```python
from build123d import *

# Parameters (mm, degrees)
SKETCH_1_R      = 3.4
SKETCH_1_W      = 10
SKETCH_1_H      = 10
EXTRUDE_1_DEPTH = 1000


with BuildPart() as part:
    # Эскиз1 → Бобышка-Вытянуть1 (new body)
    with BuildSketch(Plane.XY):
        with BuildLine():
            Line((-20, 27), (-20, 40))
            Line((-20, 40), (-7, 40))
            Line((-7, 40), (-4.1, 40))
            Line((-4.1, 40), (-4.1, 37.1))
            Line((-4.1, 37.1), (-7, 37.1))
            Line((-7, 37.1), (-7, 28.6))
            Line((-7, 28.6), (-4.582423707, 28.6))
            ThreePointArc((-4.582423707, 28.6), (-4.3976478, 28.476536686), (-4.44100235, 28.258578644))
            Line((-4.44100235, 28.258578644), (-5.571973038, 27.127607956))
            Line((-5.571973038, 27.127607956), (-2.743545913, 24.299180832))
            ThreePointArc((-2.743545913, 24.299180832), (0, 25.1), (2.743545913, 24.299180832))
            Line((2.743545913, 24.299180832), (5.571973038, 27.127607956))
            Line((5.571973038, 27.127607956), (4.44100235, 28.258578644))
            ThreePointArc((4.44100235, 28.258578644), (4.3976478, 28.476536686), (4.582423707, 28.6))
            Line((4.582423707, 28.6), (7, 28.6))
            Line((7, 28.6), (7, 37.1))
            Line((7, 37.1), (4.1, 37.1))
            Line((4.1, 37.1), (4.1, 40))
            Line((4.1, 40), (7, 40))
            Line((7, 40), (20, 40))
            Line((20, 40), (20, 27))
            Line((20, 27), (20, 24.1))
            Line((20, 24.1), (17.1, 24.1))
            Line((17.1, 24.1), (17.1, 27))
            Line((17.1, 27), (8.6, 27))
            Line((8.6, 27), (8.6, 24.582423707))
            ThreePointArc((8.6, 24.582423707), (8.476536686, 24.3976478), (8.258578644, 24.44100235))
            Line((8.258578644, 24.44100235), (7.127607956, 25.571973038))
            Line((7.127607956, 25.571973038), (4.299180832, 22.743545913))
            ThreePointArc((4.299180832, 22.743545913), (5.1, 20), (4.299180832, 17.256454087))
            Line((4.299180832, 17.256454087), (7.127607956, 14.428026962))
            Line((7.127607956, 14.428026962), (8.258578644, 15.55899765))
            ThreePointArc((8.258578644, 15.55899765), (8.476536686, 15.6023522), (8.6, 15.417576293))
            Line((8.6, 15.417576293), (8.6, 13))
            Line((8.6, 13), (17.1, 13))
            Line((17.1, 13), (17.1, 15.9))
            Line((17.1, 15.9), (20, 15.9))
            Line((20, 15.9), (20, 13))
            Line((20, 13), (20, -13))
            Line((20, -13), (20, -15.9))
            Line((20, -15.9), (17.1, -15.9))
            Line((17.1, -15.9), (17.1, -13))
            Line((17.1, -13), (8.6, -13))
            Line((8.6, -13), (8.6, -15.417576293))
            ThreePointArc((8.6, -15.417576293), (8.476536686, -15.6023522), (8.258578644, -15.55899765))
            Line((8.258578644, -15.55899765), (7.127607956, -14.428026962))
            Line((7.127607956, -14.428026962), (4.299180832, -17.256454087))
            ThreePointArc((4.299180832, -17.256454087), (5.1, -20), (4.299180832, -22.743545913))
            Line((4.299180832, -22.743545913), (7.127607956, -25.571973038))
            Line((7.127607956, -25.571973038), (8.258578644, -24.44100235))
            ThreePointArc((8.258578644, -24.44100235), (8.476536686, -24.3976478), (8.6, -24.582423707))
            Line((8.6, -24.582423707), (8.6, -27))
            Line((8.6, -27), (17.1, -27))
            Line((17.1, -27), (17.1, -24.1))
            Line((17.1, -24.1), (20, -24.1))
            Line((20, -24.1), (20, -27))
            Line((20, -27), (20, -40))
            Line((20, -40), (7, -40))
            Line((7, -40), (4.1, -40))
            Line((4.1, -40), (4.1, -37.1))
            Line((4.1, -37.1), (7, -37.1))
            Line((7, -37.1), (7, -28.6))
            Line((7, -28.6), (4.582423707, -28.6))
            ThreePointArc((4.582423707, -28.6), (4.3976478, -28.476536686), (4.44100235, -28.258578644))
            Line((4.44100235, -28.258578644), (5.571973038, -27.127607956))
            Line((5.571973038, -27.127607956), (2.743545913, -24.299180832))
            ThreePointArc((2.743545913, -24.299180832), (0, -25.1), (-2.743545913, -24.299180832))
            Line((-2.743545913, -24.299180832), (-5.571973038, -27.127607956))
            Line((-5.571973038, -27.127607956), (-4.44100235, -28.258578644))
            ThreePointArc((-4.44100235, -28.258578644), (-4.3976478, -28.476536686), (-4.582423707, -28.6))
            Line((-4.582423707, -28.6), (-7, -28.6))
            Line((-7, -28.6), (-7, -37.1))
            Line((-7, -37.1), (-4.1, -37.1))
            Line((-4.1, -37.1), (-4.1, -40))
            Line((-4.1, -40), (-7, -40))
            Line((-7, -40), (-20, -40))
            Line((-20, -40), (-20, -27))
            Line((-20, -27), (-20, -24.1))
            Line((-20, -24.1), (-17.1, -24.1))
            Line((-17.1, -24.1), (-17.1, -27))
            Line((-17.1, -27), (-8.6, -27))
            Line((-8.6, -27), (-8.6, -24.582423707))
            ThreePointArc((-8.6, -24.582423707), (-8.476536686, -24.3976478), (-8.258578644, -24.44100235))
            Line((-8.258578644, -24.44100235), (-7.127607956, -25.571973038))
            Line((-7.127607956, -25.571973038), (-4.299180832, -22.743545913))
            ThreePointArc((-4.299180832, -22.743545913), (-5.1, -20), (-4.299180832, -17.256454087))
            Line((-4.299180832, -17.256454087), (-7.127607956, -14.428026962))
            Line((-7.127607956, -14.428026962), (-8.258578644, -15.55899765))
            ThreePointArc((-8.258578644, -15.55899765), (-8.476536686, -15.6023522), (-8.6, -15.417576293))
            Line((-8.6, -15.417576293), (-8.6, -13))
            Line((-8.6, -13), (-17.1, -13))
            Line((-17.1, -13), (-17.1, -15.9))
            Line((-17.1, -15.9), (-20, -15.9))
            Line((-20, -15.9), (-20, -13))
            Line((-20, -13), (-20, 13))
            Line((-20, 13), (-20, 15.9))
            Line((-20, 15.9), (-17.1, 15.9))
            Line((-17.1, 15.9), (-17.1, 13))
            Line((-17.1, 13), (-8.6, 13))
            Line((-8.6, 13), (-8.6, 15.417576293))
            ThreePointArc((-8.6, 15.417576293), (-8.476536686, 15.6023522), (-8.258578644, 15.55899765))
            Line((-8.258578644, 15.55899765), (-7.127607956, 14.428026962))
            Line((-7.127607956, 14.428026962), (-4.299180832, 17.256454087))
            ThreePointArc((-4.299180832, 17.256454087), (-5.1, 20), (-4.299180832, 22.743545913))
            Line((-4.299180832, 22.743545913), (-7.127607956, 25.571973038))
            Line((-7.127607956, 25.571973038), (-8.258578644, 24.44100235))
            ThreePointArc((-8.258578644, 24.44100235), (-8.476536686, 24.3976478), (-8.6, 24.582423707))
            Line((-8.6, 24.582423707), (-8.6, 27))
            Line((-8.6, 27), (-17.1, 27))
            Line((-17.1, 27), (-17.1, 24.1))
            Line((-17.1, 24.1), (-20, 24.1))
            Line((-20, 24.1), (-20, 27))
        make_face()
        with Locations((0, 20)):
            Circle(SKETCH_1_R, mode=Mode.SUBTRACT)
        with Locations((0, -20)):
            Circle(SKETCH_1_R, mode=Mode.SUBTRACT)
        with Locations((13.5, 33.5)):
            Rectangle(SKETCH_1_W, SKETCH_1_H, mode=Mode.SUBTRACT)
        with Locations((-13.5, 33.5)):
            Rectangle(SKETCH_1_W, SKETCH_1_H, mode=Mode.SUBTRACT)
        with Locations((13.5, -33.5)):
            Rectangle(SKETCH_1_W, SKETCH_1_H, mode=Mode.SUBTRACT)
        with Locations((-13.5, -33.5)):
            Rectangle(SKETCH_1_W, SKETCH_1_H, mode=Mode.SUBTRACT)
        with BuildLine():
            Line((-17.7, 11.5), (-7.085786438, 11.5))
            Line((-7.085786438, 11.5), (-2.829134161, 15.756652277))
            ThreePointArc((-2.829134161, 15.756652277), (0, 14.9), (2.829134161, 15.756652277))
            Line((2.829134161, 15.756652277), (7.085786438, 11.5))
            Line((7.085786438, 11.5), (17.7, 11.5))
            ThreePointArc((17.7, 11.5), (18.265685425, 11.265685425), (18.5, 10.7))
            Line((18.5, 10.7), (18.5, -10.7))
            ThreePointArc((18.5, -10.7), (18.265685425, -11.265685425), (17.7, -11.5))
            Line((17.7, -11.5), (7.085786438, -11.5))
            Line((7.085786438, -11.5), (2.829134161, -15.756652277))
            ThreePointArc((2.829134161, -15.756652277), (0, -14.9), (-2.829134161, -15.756652277))
            Line((-2.829134161, -15.756652277), (-7.085786438, -11.5))
            Line((-7.085786438, -11.5), (-17.7, -11.5))
            ThreePointArc((-17.7, -11.5), (-18.265685425, -11.265685425), (-18.5, -10.7))
            Line((-18.5, -10.7), (-18.5, 10.7))
            ThreePointArc((-18.5, 10.7), (-18.265685425, 11.265685425), (-17.7, 11.5))
        make_face(mode=Mode.SUBTRACT)
    extrude(amount=EXTRUDE_1_DEPTH)


solid = part.part
```
The listing builds one solid part. Answer for the finished solid, in the listing's coordinates (mm). A direction names the side the tool comes from. Give positions to 0.01 mm unless a question says otherwise; leave off trailing zeros. Order: outer loops, then holes, each group sorted by start corner. A loop starts at its lowest first (then second) coordinate and runs counter-clockwise, first axis right, second up. Notation, with made-up numbers: M 4,47.5 L 10,47.5 A29 ccw 10,74.5 Z; hole C -3.75,-28 d5. An arc over 180 degrees is marked long. Put each result on its own line as item: value. Start each with the question number.
Item 1: Which of the six approach directions +Z, -Z, +X, -X, +Y, -Y give full straight-line access (tool end or side, diameter ignored) to faces 4 (the face through (20, 0, 493)), 5 (the face through (18.5, 0, 493))?
Item 2: The part is cut by section B-B, the plane z = 263.5. State how many separate pieces and enclosed holes the cut face has, and give its area (3 significant figures).
Item 3: Find the intervals of material crossed by line 1 along X through (y, z) = (29, 150); line 2 along Y through (x, z) = (-1, 304.5); line 3 along Y through (x, z) = (16, 519.5), in increasing order.
Item 4: For a pull along X with two mould halves and no side action, classify faces 1 (the face through (-7, 12, 1000)), 2 (the face through (-20, -32, 493)), 3 (the face through (-18.5, 0, 493)) as +X half, -X half, draft (parallel to the pull), parting line (faces both ways), or undercut.
Item 5: The part is cut by section A-A, the plane y = 0. Determine the outline of the cut face in (x, z).
Answer key:
1. face 4: +Z, -Z, +X, +Y, -Y
1. face 5: +Z, -Z
2. separate pieces: 1
2. enclosed holes: 7
2. area: 733 mm²
3. line 1: x = -20 to -18.5, -8.5 to -7, 7 to 8.5, 18.5 to 20
3. line 2: y = -25 to -23.25, -16.75 to -15, 15 to 16.75, 23.25 to 25
3. line 3: y = -40 to -38.5, -28.5 to -27, -13 to -11.5, 11.5 to 13, 27 to 28.5, 38.5 to 40
4. face 1: draft
4. face 2: -X half
4. face 3: undercut
5. outline: M -20,0 L -18.5,0 L -18.5,1000 L -20,1000 Z; M 18.5,0 L 20,0 L 20,1000 L 18.5,1000 Z
